The model under review builds one solid part; all positions refer to its coordinate system, in mm. A direction names the side the tool comes from. Coordinates: 2 decimals unless noted, no trailing zeros. Loops run counter-clockwise (first coordinate to the right, second up) from the corner with the lowest first, then second, coordinate; pieces in that order, holes last. Notation, with made-up numbers: M 45.25,66.25 L 75.25,66.25 A12 ccw 75.25,75.25 Z; hole C 4,17 d2. An arc over 180 degrees is marked long. Write item = value, one per line. Start each with the question number.
Q1. Mouldability with a two-part tool opening along Z and no side actions: class faces 3 (the face through (5.5, 2, -37)), 4 (the face through (18.122, 1.479, -30.864)), 5 (the face through (-9, 1, -33)), 6 (the face through (4.5, 1, -35)) as released by +Z, released by -Z, zero draft, split by the parting line, or undercut.
Q2. We need section D-D on z = -5.5. Give the boundary of the cut face in (x, y), and give its area (3 significant figures).
Q3. Clearance check with flat-ended pins moving along their axes: pin 1 Ø1.5 at (x, y) = (-8.5, 1) entering from +Z; pin 2 Ø1.2 at (y, z) = (2, -34) entering from -X; pin 3 Ø1 at (x, y) = (12, 1.5) entering from +Z. State where each tip first meets the part, or that it passes through.
Q4. We need section B-B on z = -19. Give the boundary of the cut face in (x, y).
Q5. We need section A-A on y = 1.7. Give the boundary of the cut face in (x, z), and give its area (3 significant figures).
Q6. Wall thickness on probe 1 along Z at (x, y) = (-10, 2.1); probe 2 along X at (y, z) = (0.9, -33); probe 3 along Z at (x, y) = (0, 1.05): over which ranges is each line inside the solid? List them lowest first.
Q7. For faces 1 (the face through (-4.5, 1, -41)), 2 (the face through (0, 3, -29)), list the 3-axis set-ups (+Z, -Z, +X, -X, +Y, -Y) from which the entire face can be reached by the end or side of a thin tool; tool diameter is ignored.
Q8. We need section C-C on z = -33. Give the boundary of the cut face in (x, y).
from build123d import *

# Parameters (mm, degrees)
BOSS_EXTRUDE1_DEPTH     = 1
BOSS_EXTRUDE2_DEPTH     = 2
SKETCH5_R               = 2.25
SKETCH5_R_2             = 0.5
CUT_EXTRUDE2_DEPTH      = 75.390311459
CUT_EXTRUDE3_DEPTH      = 75.423910398
CUT_EXTRUDE3_DEPTH_BACK = 75.423910398
SKETCH6_OUTSIDE_W       = 86.15
SKETCH6_OUTSIDE_H       = 123.471
SKETCH6_OUTSIDE_R       = 30.5
BOSS_EXTRUDE3_DEPTH     = 3
SKETCH8_W               = 9
SKETCH8_H               = 28.4
CUT_EXTRUDE4_DEPTH      = 3
SKETCH10_W              = 0.894041394
SKETCH10_H              = 3.5
SKETCH10_W_2            = 1
CUT_EXTRUDE6_DEPTH      = 13
CUT_EXTRUDE7_DEPTH      = 57.949539067
CUT_EXTRUDE7_DEPTH_BACK = 57.949539067
SKETCH11_R              = 27.5
SKETCH11_W              = 9
SKETCH11_H              = 14.2
CUT_EXTRUDE8_DEPTH      = 57.949539067
CUT_EXTRUDE8_DEPTH_BACK = 57.949539067
SKETCH12_R              = 1


with BuildPart() as part:
    # Sketch2 → Boss-Extrude1 (new body)
    with BuildSketch(Plane(origin=(0, 0, 0), x_dir=(1, 0, 0), z_dir=(0, 1, 0))):
        with BuildLine():
            Line((-9.5, 67.820855486), (9.5, 67.820855486))
            ThreePointArc((9.5, 67.820855486), (11.621320344, 66.94217583), (12.5, 64.820855486))
            Line((12.5, 64.820855486), (12.5, 33.674916481))
            ThreePointArc((12.5, 33.674916481), (13.680828963, 28.960871273), (16.944444444, 25.360122288))
            ThreePointArc((16.944444444, 25.360122288), (0, -30.5), (-16.944444444, 25.360122288))
            ThreePointArc((-16.944444444, 25.360122288), (-13.680828963, 28.960871273), (-12.5, 33.674916481))
            Line((-12.5, 33.674916481), (-12.5, 64.820855486))
            ThreePointArc((-12.5, 64.820855486), (-11.621320344, 66.94217583), (-9.5, 67.820855486))
        make_face()
        with BuildLine():
            Line((3.5516796, -15.713533545), (4.759805249, -3.321913887))
            Line((4.759805249, -3.321913887), (6.334764225, -3.329153378))
            ThreePointArc((6.334764225, -3.329153378), (9.649898055, -0.044356931), (6.365101608, 3.270776898))
            Line((6.365101608, 3.270776898), (4.790142632, 3.278016389))
            Line((4.790142632, 3.278016389), (3.695984805, 15.680218773))
            ThreePointArc((3.695984805, 15.680218773), (0.087334891, 18.999799278), (-3.5516796, 15.713533545))
            Line((-3.5516796, 15.713533545), (-4.759805249, 3.321913887))
            Line((-4.759805249, 3.321913887), (-6.334764225, 3.329153378))
            ThreePointArc((-6.334764225, 3.329153378), (-9.649898055, 0.044356931), (-6.365101608, -3.270776898))
            Line((-6.365101608, -3.270776898), (-4.790142632, -3.278016389))
            Line((-4.790142632, -3.278016389), (-3.695984805, -15.680218773))
            ThreePointArc((-3.695984805, -15.680218773), (-0.087334891, -18.999799278), (3.5516796, -15.713533545))
        make_face(mode=Mode.SUBTRACT)
    extrude(amount=BOSS_EXTRUDE1_DEPTH)

    # Sketch3 → Boss-Extrude2 (add)
    with BuildSketch(Plane(origin=(0, 1, 0), x_dir=(1, 0, 0), z_dir=(0, 1, 0))):
        with BuildLine():
            Line((-12.5, 64.820855486), (-12.5, 33.674916481))
            ThreePointArc((-12.5, 33.674916481), (-13.680828963, 28.960871273), (-16.944444444, 25.360122288))
            ThreePointArc((-16.944444444, 25.360122288), (0, -30.5), (16.944444444, 25.360122288))
            ThreePointArc((16.944444444, 25.360122288), (13.680828963, 28.960871273), (12.5, 33.674916481))
            Line((12.5, 33.674916481), (12.5, 64.820855486))
            ThreePointArc((12.5, 64.820855486), (11.621320344, 66.94217583), (9.5, 67.820855486))
            Line((9.5, 67.820855486), (-9.5, 67.820855486))
            ThreePointArc((-9.5, 67.820855486), (-11.621320344, 66.94217583), (-12.5, 64.820855486))
        make_face()
    extrude(amount=BOSS_EXTRUDE2_DEPTH)

    # Sketch5 → Cut-Extrude2 (cut, through all)
    with BuildSketch(Plane.XZ.offset(-1)):
        with Locations(Location((0, 0, 0), (0, 0, 270))):
            Circle(SKETCH5_R)
        with Locations(Location((0.022708028, 13.233852211, 0), (0, 0, 270))):
            Circle(SKETCH5_R_2)
        with Locations(Location((-6.853849078, 0.011760551, 0), (0, 0, 270))):
            Circle(SKETCH5_R_2)
        with Locations(Location((-0.022708028, -13.233852211, 0), (0, 0, 270))):
            Circle(SKETCH5_R_2)
        with Locations(Location((6.853849078, -0.011760551, 0), (0, 0, 270))):
            Circle(SKETCH5_R_2)
    extrude(amount=-CUT_EXTRUDE2_DEPTH, mode=Mode.SUBTRACT)

    # Sketch6 outside → Cut-Extrude3 (cut, two sides: drawn at the far end of the back side and taken through both)
    with BuildSketch(Plane(origin=(0, 3, 0), x_dir=(1, 0, 0), z_dir=(0, 1, 0)).offset(-CUT_EXTRUDE3_DEPTH_BACK)):
        with Locations((0, 18.6605)):
            Rectangle(SKETCH6_OUTSIDE_W, SKETCH6_OUTSIDE_H)
        with Locations(Location((0, 0, 0), (0, 0, 270))):
            Circle(SKETCH6_OUTSIDE_R, mode=Mode.SUBTRACT)
    extrude(amount=CUT_EXTRUDE3_DEPTH + CUT_EXTRUDE3_DEPTH_BACK, mode=Mode.SUBTRACT)

    # Sketch7 → Boss-Extrude3 (add)
    with BuildSketch(Plane.XZ):
        with BuildLine():
            Line((-7.798950698, -48), (7.798950698, -48))
            ThreePointArc((7.798950698, -48), (8.828603574, -47.714588859), (9.564382048, -46.939814955))
            Line((9.564382048, -46.939814955), (26.92282808, -14.332178068))
            Line((26.92282808, -14.332178068), (0, -22.549328153))
            Line((0, -22.549328153), (-26.92282808, -14.332178068))
            Line((-26.92282808, -14.332178068), (-9.564382048, -46.939814955))
            ThreePointArc((-9.564382048, -46.939814955), (-8.828603574, -47.714588859), (-7.798950698, -48))
        make_face()
    extrude(amount=-BOSS_EXTRUDE3_DEPTH)

    # Sketch8 → Cut-Extrude4 (cut)
    with BuildSketch(Plane.XZ):
        with Locations((0, -48)):
            Rectangle(SKETCH8_W, SKETCH8_H)
    extrude(amount=-CUT_EXTRUDE4_DEPTH, mode=Mode.SUBTRACT)

    # Sketch10 → Cut-Extrude6 (cut)
    with BuildSketch(Plane.XZ.offset(-3)):
        with Locations((4.052979303, -37.05)):
            Rectangle(SKETCH10_W, SKETCH10_H)
        with Locations((5, -37.05)):
            Rectangle(SKETCH10_W_2, SKETCH10_H)
    extrude(amount=CUT_EXTRUDE6_DEPTH, mode=Mode.SUBTRACT)

    # Sketch11 → Cut-Extrude7 (cut, two sides: drawn at the far end of the back side and taken through both)
    with BuildSketch(Plane.XZ.offset(-CUT_EXTRUDE7_DEPTH_BACK)):
        with Locations(Location((0, 0, 0), (0, 0, 270))):
            Circle(SKETCH11_R)
        with Locations((0, -40.9)):
            Rectangle(SKETCH11_W, SKETCH11_H)
    extrude(amount=CUT_EXTRUDE7_DEPTH + CUT_EXTRUDE7_DEPTH_BACK, mode=Mode.SUBTRACT)

    # Sketch12 → Cut-Extrude8 (cut, two sides: drawn at the far end of the back side and taken through both)
    with BuildSketch(Plane(origin=(0, 3, 0), x_dir=(1, 0, 0), z_dir=(0, 1, 0)).offset(-CUT_EXTRUDE8_DEPTH_BACK)):
        with Locations(Location((-10, 33, 0), (0, 0, 270))):
            Circle(SKETCH12_R)
        with Locations(Location((10, 33, 0), (0, 0, 270))):
            Circle(SKETCH12_R)
    extrude(amount=CUT_EXTRUDE8_DEPTH + CUT_EXTRUDE8_DEPTH_BACK, mode=Mode.SUBTRACT)


solid = part.part
Returned:
q1.face_3 = undercut
q1.face_4 = released by -Z
q1.face_5 = undercut
q1.face_6 = zero draft
q2.outline = M -30,0 L -26.94,0 L -26.94,3 L -30,3 Z; M 26.94,0 L 30,0 L 30,3 L 26.94,3 Z
q2.area = 18.3 mm^2
q3.pin_1 = 29.5
q3.pin_2 = -16.77
q3.pin_3 = 28.25
q4.outline = M -24.44,0 L -19.88,0 L -19.88,3 L -24.44,3 Z; M 19.88,0 L 24.44,0 L 24.44,3 L 19.88,3 Z
q5.outline = M -26.92,-14.33 L -9.56,-46.94 A2 ccw -7.8,-48 L -4.5,-48 L -4.5,-33.8 L 4.5,-33.8 L 4.5,-35.3 L 5.5,-35.3 L 5.5,-38.8 L 4.5,-38.8 L 4.5,-48 L 7.8,-48 A2 ccw 9.56,-46.94 L 26.92,-14.33 A30.5 ccw long Z; hole C 0,0 d55; hole C -10,-33 d2; hole C 10,-33 d2
q5.area = 998 mm^2
q6.probe_1 = -46.12 to -34, -32 to -25.62, 25.62 to 28.81
q6.probe_2 = -16.99 to -11, -9 to 9, 11 to 16.99
q6.probe_3 = -33.8 to -27.5, 27.5 to 30.5
q7.face_1 = -Z, +Y, -Y
q7.face_2 = +Z, -Z, +X, -X, +Y
q8.outline = M -16.99,0 L -11,0 L -11,3 L -16.99,3 Z; M -9,0 L 9,0 L 9,3 L -9,3 Z; M 11,0 L 16.99,0 L 16.99,3 L 11,3 Z
